The listing builds one solid part. Answer for the finished solid, in the listing's coordinates (mm). Face numbers are marked on the shaded views. A direction names the side the tool comes from. Give positions to 0.01 mm unless a question says otherwise; leave off trailing zeros. Write each loop counter-clockwise with the first axis right and the second up, starting at its lowest first coordinate (ties: lowest second). Pieces come first, ordered by that corner, then holes. Notation, with made-up numbers: (33.5, -36) -> (39.5, -36) arc R36 cw to (39.5, -2) -> close; hole circle Ø4 at (24.5, 60.25). An arc over 180 degrees is marked (long way). Put each result on its own line as item: value. Start each with the question number.
1) Flat-ended cylindrical pins translate along their axes: pin 1 Ø1 at (y, z) = (2.5, -3.5) entering from +X; pin 2 Ø3 at (x, z) = (-11.5, -3) entering from -Y; pin 3 Ø5 at (x, z) = (-29.5, 4.5) entering from +Y. Find the tip coordinate at first contact, or state that the pin passes through.
2) Find the intervals of material crossed by line 1 along X through (y, z) = (1.5, 3.5); line 2 along X through (y, z) = (5.25, 4); line 3 along Z through (x, y) = (5.5, 5.25), in increasing order. Write a range as from..to.
3) A cutting plane is placed at C-C (y = 0.5). Write down the section's boundary in (x, z) (3 decimals), then the cut area to 3 significant figures.
4) A cutting plane is placed at A-A (x = 1). Write down the section's boundary in (y, z) (3 decimals), then the cut area to 3 significant figures.
5) A cutting plane is placed at D-D (x = -27). Write down the section's boundary in (y, z) (3 decimals).
6) A cutting plane is placed at B-B (z = 1.75). Write down the section's boundary in (x, y) (3 decimals).
7) For the marked faces 1 and 2, determine the directions among +Z, -Z, +X, -X, +Y, -Y from which every point of the face is accessible in a straight line to the end or side of a thin tool.
from build123d import *

# Parameters (mm, degrees)
BOSS_EXTRUDE1_DEPTH = 6.35
SKETCH2_R           = 3.175
BOSS_EXTRUDE2_DEPTH = 25.4


with BuildPart() as part:
    # Sketch1 → Boss-Extrude1 (new body)
    with BuildSketch(Plane(origin=(0, 0, 0), x_dir=(1, 0, 0), z_dir=(0, 1, 0))):
        with BuildLine():
            Line((-8.980256121, 3.175), (-8.980256121, -3.175))
            ThreePointArc((-8.980256121, -3.175), (9.525, 0), (-8.980256121, 3.175))
        make_face()
    extrude(amount=BOSS_EXTRUDE1_DEPTH)

    # Sketch2 → Boss-Extrude2 (add)
    with BuildSketch(Plane.ZY.offset(8.980256121)):
        with Locations((0, 3.175)):
            Circle(SKETCH2_R)
    extrude(amount=BOSS_EXTRUDE2_DEPTH)

    # Sketch3 → Cut-Revolve1 (revolve, cut)
    with BuildSketch(Plane.XY):
        with BuildLine():
            Line((0, 9.525), (0, -3.175))
            ThreePointArc((0, -3.175), (6.35, 3.175), (0, 9.525))
        make_face()
    revolve(axis=Axis((0, 6.35, 0), (0, -1, 0)), mode=Mode.SUBTRACT)


solid = part.part
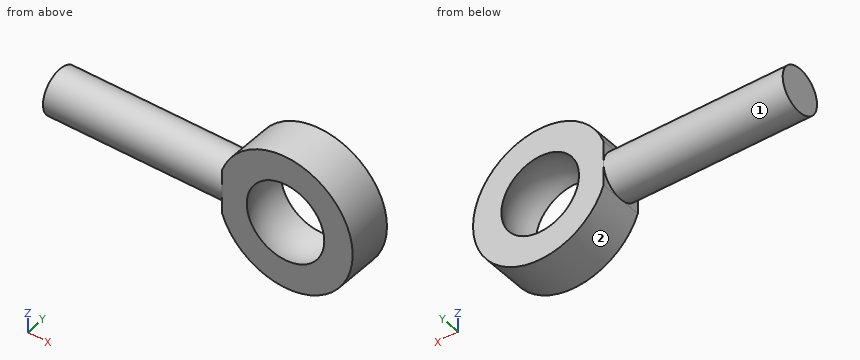
Reply:
1. pin 1: stops at x = 9.04
1. pin 2: stops at y = 0.38
1. pin 3: stops at y = 5.64
2. line 1: x = -8.86..-5.03, 5.03..8.86
2. line 2: x = -8.64..-4.47, 4.47..8.64
2. line 3: z = -7.78..-2.4, 2.4..7.78
3. outline: (-34.38, -1.71) -> (-8.98, -1.71) -> (-8.98, -3.175) arc R9.525 ccw (long way) to (-8.98, 3.175) -> (-8.98, 1.71) -> (-34.38, 1.71) -> close; hole circle Ø11.518 at (0, 0)
3. area: 265 mm2
4. outline: (0, -9.472) -> (6.35, -9.472) -> (6.35, -5.408) arc R6.271 cw to (0, -5.408) -> close; (0, 5.408) arc R6.271 cw to (6.35, 5.408) -> (6.35, 9.472) -> (0, 9.472) -> close
4. area: 44.2 mm2
5. outline: circle Ø6.35 at (3.175, 0)
6. outline: (-34.38, 0.526) -> (-8.98, 0.526) -> (-8.98, 0) -> (-5.213, 0) arc R6.104 cw to (-5.213, 6.35) -> (-8.98, 6.35) -> (-8.98, 5.824) -> (-34.38, 5.824) -> close; (5.213, 0) -> (9.363, 0) -> (9.363, 6.35) -> (5.213, 6.35) arc R6.104 cw to start
7. face 1: -X
7. face 2: +Y, -Y
